from build123d import *

# Parameters (mm, degrees)
BOSS_EXTRUDE1_DEPTH = 5
SKETCH2_R           = 1.5
CUT_EXTRUDE1_DEPTH  = 10
SKETCH3_W           = 10
SKETCH3_H           = 5
SKETCH3_W_2         = 5
SKETCH3_H_2         = 10
CUT_EXTRUDE2_DEPTH  = 10
SKETCH4_R           = 1.5
SKETCH4_W           = 15
SKETCH4_H           = 20
CUT_EXTRUDE3_DEPTH  = 10
SKETCH5_R           = 1.5
CUT_EXTRUDE4_DEPTH  = 10


with BuildPart() as part:
    # Sketch1 → Boss-Extrude1 (new body)
    with BuildSketch(Plane(origin=(0, 0, 0), x_dir=(1, 0, 0), z_dir=(0, 1, 0))):
        with BuildLine():
            Line((-45, 110), (45, 110))
            Line((45, 110), (45, 143.090880213))
            ThreePointArc((45, 143.090880213), (129.903810568, 75), (146.420337314, -32.574296936))
            Line((146.420337314, -32.574296936), (117.762794416, -16.02885683))
            Line((117.762794416, -16.02885683), (72.762794416, -93.97114317))
            Line((72.762794416, -93.97114317), (101.420337314, -110.516583277))
            ThreePointArc((101.420337314, -110.516583277), (0, -150), (-101.420337314, -110.516583277))
            Line((-101.420337314, -110.516583277), (-72.762794416, -93.97114317))
            Line((-72.762794416, -93.97114317), (-117.762794416, -16.02885683))
            Line((-117.762794416, -16.02885683), (-146.420337314, -32.574296936))
            ThreePointArc((-146.420337314, -32.574296936), (-129.903810568, 75), (-45, 143.090880213))
            Line((-45, 143.090880213), (-45, 110))
        make_face()
    extrude(amount=BOSS_EXTRUDE1_DEPTH)

    # Sketch2 → Cut-Extrude1 (cut)
    with BuildSketch(Plane(origin=(0, 5, 0), x_dir=(1, 0, 0), z_dir=(0, 1, 0))):
        with Locations(Location((-10, 95, 0), (0, 0, 270))):
            Circle(SKETCH2_R)
        with Locations(Location((10, 95, 0), (0, 0, 270))):
            Circle(SKETCH2_R)
        with Locations(Location((-87.27241336, -38.839745962, 0), (0, 0, 270))):
            Circle(SKETCH2_R)
        with Locations(Location((-77.27241336, -56.160254038, 0), (0, 0, 270))):
            Circle(SKETCH2_R)
        with Locations(Location((77.27241336, -56.160254038, 0), (0, 0, 270))):
            Circle(SKETCH2_R)
        with Locations(Location((87.27241336, -38.839745962, 0), (0, 0, 270))):
            Circle(SKETCH2_R)
    extrude(amount=-CUT_EXTRUDE1_DEPTH, mode=Mode.SUBTRACT)

    # Sketch3 → Cut-Extrude2 (cut)
    with BuildSketch(Plane(origin=(0, 5, 0), x_dir=(1, 0, 0), z_dir=(0, 1, 0))):
        with Locations((45, 87.5)):
            Rectangle(SKETCH3_W, SKETCH3_H)
        with Locations((-45, 87.5)):
            Rectangle(SKETCH3_W, SKETCH3_H)
        with Locations((-73.5, 45)):
            Rectangle(SKETCH3_W_2, SKETCH3_H_2)
        with Locations((73.5, 45)):
            Rectangle(SKETCH3_W_2, SKETCH3_H_2)
        with Locations((-45, -40.5)):
            Rectangle(SKETCH3_W, SKETCH3_H)
        with Locations((45, -40.5)):
            Rectangle(SKETCH3_W, SKETCH3_H)
        with Locations((-70.5, -10)):
            Rectangle(SKETCH3_W_2, SKETCH3_H_2)
        with Locations((70.5, -10)):
            Rectangle(SKETCH3_W_2, SKETCH3_H_2)
    extrude(amount=-CUT_EXTRUDE2_DEPTH, mode=Mode.SUBTRACT)

    # Sketch4 → Cut-Extrude3 (cut)
    with BuildSketch(Plane(origin=(0, 5, 0), x_dir=(1, 0, 0), z_dir=(0, 1, 0))):
        with Locations(Location((-15.25, -63, 0), (0, 0, 270))):
            Circle(SKETCH4_R)
        with Locations(Location((15.25, -63, 0), (0, 0, 270))):
            Circle(SKETCH4_R)
        with Locations(Location((-15.25, -93.5, 0), (0, 0, 270))):
            Circle(SKETCH4_R)
        with Locations(Location((15.25, -93.5, 0), (0, 0, 270))):
            Circle(SKETCH4_R)
        with Locations((-37.75, -78.25)):
            Rectangle(SKETCH4_W, SKETCH4_H)
    extrude(amount=-CUT_EXTRUDE3_DEPTH, mode=Mode.SUBTRACT)

    # Sketch5 → Cut-Extrude4 (cut)
    with BuildSketch(Plane(origin=(0, 5, 0), x_dir=(1, 0, 0), z_dir=(0, 1, 0))):
        with Locations(Location((-112.583302492, 65, 0), (0, 0, 270))):
            Circle(SKETCH5_R)
        with Locations(Location((112.583302492, 65, 0), (0, 0, 270))):
            Circle(SKETCH5_R)
        with Locations(Location((0, -130, 0), (0, 0, 270))):
            Circle(SKETCH5_R)
    extrude(amount=-CUT_EXTRUDE4_DEPTH, mode=Mode.SUBTRACT)


solid = part.part
Build history of the part. All positions in model axes, mm. A direction names the side the tool comes from. Round coordinates to 2 decimals unless told otherwise and drop trailing zeros. Write each loop counter-clockwise with the first axis right and the second up, starting at its lowest first coordinate (ties: lowest second). Pieces come first, ordered by that corner, then holes. Notation, with made-up numbers: (26.25, -3) -> (73.25, -3) arc R31 cw to (73.25, 36) -> close; hole circle Ø10 at (-13, 73). An arc over 180 degrees is marked (long way). Use one line per item in the form item = value.
Q1. Band-saw the part on A-A, the plane z = 83. Write the cut outline in (x, y).
Conclusion:
outline = (-79.1, 0) -> (-45.25, 0) -> (-45.25, 5) -> (-79.1, 5) -> close; (-30.25, 0) -> (79.1, 0) -> (79.1, 5) -> (-30.25, 5) -> close
Q2. Band-saw the part on B-B, the plane y = 3.4. State how many separate pieces and enclosed holes the cut face has, then the cut area to 3 significant figures.
Conclusion:
separate_pieces = 1
enclosed_holes = 22
area = 59,700 mm²
Q3. Drill centre lines: L1, parallel to X at y = 2.4, z = 93.5; L2, parallel to X at y = 2.3, z = 38.5; L3, parallel to X at y = 2.15, z = 63. Where is each one in solid material? Low to high.
Conclusion:
L1 = -73.03 to -16.75, -13.75 to 13.75, 16.75 to 73.03
L2 = -104.79 to -88.73, -85.81 to -50, -40 to 40, 50 to 85.81, 88.73 to 104.79
L3 = -90.64 to -16.75, -13.75 to 13.75, 16.75 to 90.64
Q4. Two-plate mould, pull along X, no slides. Class faces 6 (the flat face through (-94.948, 2.465, 55.546)), 7 (the flat face through (2, 0, 1)), 8 (the cylindrical face through (129.117, 2.465, -76.346)): released by +X, released by -X, zero draft, split by the parting line, or undercut.
Conclusion:
face_6 = undercut
face_7 = zero draft
face_8 = released by +X
Q5. Drop flat-ended pins along their axis: P1, Ø1.5, axis at y = 2.5, z = 81, coming from the -X side; P2, Ø2, axis at y = 4.5, z = 77, coming from the -X side; P3, Ø1.5, axis at x = -44, y = 2.5, coming from the +Z side; P4, Ø2.5, axis at x = -87.27, z = 38.84, coming from the +Y side. Give the stop position or say it passes through.
Conclusion:
P1 = -80.68
P2 = -83.14
P3 = 143.63
P4 = through
Q6. Band-saw the part on C-C, the plane x = -124. Write the cut outline in (y, z).
Conclusion:
outline = (0, -84.4) -> (5, -84.4) -> (5, 19.63) -> (0, 19.63) -> close
Q7. Band-saw the part on D-D, the plane z = -31.5. Write the cut outline in (x, y).
Conclusion:
outline = (-146.66, 0) -> (146.66, 0) -> (146.66, 5) -> (-146.66, 5) -> close
Q8. Tool access for faces 1 (the flat face through (-87.29, 2.46, 102.36)), 2 (the flat face through (2, 5, 1)), 3 (the flat face through (95.58, 2.46, 54.45)), 4 (the flat face through (-131.891, 2.465, 24.186)), 5 (the flat face through (86.891, 2.465, 102.128)): list every direction of +Z, -Z, +X, -X, +Y, -Y with a clear straight run to the whole face (end or side of a thin tool).
Conclusion:
face_1 = -X, +Y, -Y
face_2 = +Z, -Z, +X, -X, +Y
face_3 = +Y, -Y
face_4 = +Z, +Y, -Y
face_5 = +X, +Y, -Y
